Input: part model. Units: mm. Frame: model coordinates. Face numbers are marked on the shaded views. A direction names the side the tool comes from. Round coordinates to 2 decimals unless told otherwise and drop trailing zeros. Order: outer loops, then holes, each group sorted by start corner. A loop starts at its lowest first (then second) coordinate and runs counter-clockwise, first axis right, second up.
Item 1: First-contact query: pin 1 (0.9 mm diameter, centred on y = 6.5, z = 43, fed in from -X); pin 2 (2.5 mm diameter, centred on x = 0.5, z = 42.5, fed in from +Y); pin 3 (10 mm diameter, centred on x = -15, y = -23.5, fed in from +Z). Flat tips, straight axial feed; report the tip coordinate or a pass-through.
Item 2: Cut plane A-A on x = 27. Output: boundary loops of the cut face in (y, z), then the cut area to 3 significant figures.
Item 3: Cut plane B-B on y = 0. Output: boundary loops of the cut face in (x, z).
Item 4: Cut plane C-C on z = 12. Output: boundary loops of the cut face in (x, y).
Item 5: Mould query, pull axis Z, two halves, no side actions, for the marked faces 1, 2 and 3. Classes: released by +Z, released by -Z, zero draft, split by the parting line, or undercut.
Item 6: Reachability of the marked faces 4 and 5 from +Z, -Z, +X, -X, +Y, -Y: full face, straight path, thin tool, end or side. Return the list, or none.
Item 7: Cut plane D-D on y = 11. Output: boundary loops of the cut face in (x, z).
Item 8: Line query: L1, parallel to X at y = 0, z = -6.5; L2, parallel to X at y = 0, z = 31.5; L3, parallel to Y at x = 0, z = 41. Output: solid intervals per line, ascending.
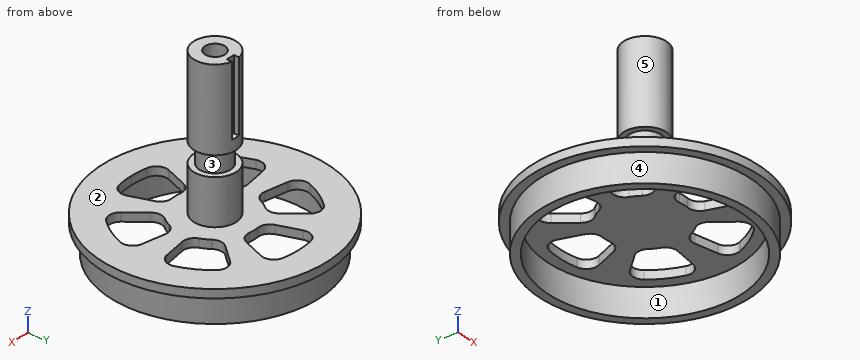
Autodesk Fusion 360 part; units mm, degrees
sketch "Sketch1" plane through (0, 0, 0) normal (0, 0, 1) x (1, 0, 0)
  circle A0 centre (0, 0) radius 33.9
  circle A1 centre (0, 0) radius 36.9
  circle A2 centre (0, 0) radius 39.9
  circle A3 centre (0, 0) radius 7.5
  circle A4 centre (0, 0) radius 14
  line L0 (0, 0) -> (4.7883, -13.1557)
  line L1 (0, 0) -> (-4.7883, -13.1557)
  line L2 (0, -60) -> (0, 60)
  line L3 (4.7883, -13.1557) -> (10.2606, -28.1908)
  line L4 (-4.7883, -13.1557) -> (-10.2606, -28.1908)
  arc A5 (10.2606, -28.1908) -> (-10.2606, -28.1908) centre (0, 0) ccw
  arc A6 (-10.2606, -28.1908) -> (0, -30) centre (0, 0) ccw
  arc A7 (0, -30) -> (10.2606, -28.1908) centre (0, 0) ccw
  line L5 (13.7873, -2.4311) -> (29.5442, -5.2094)
  line L6 (8.999, -10.7246) -> (19.2836, -22.9813)
  line L7 (8.999, 10.7246) -> (19.2836, 22.9813)
  line L8 (13.7873, 2.4311) -> (29.5442, 5.2094)
  line L9 (-4.7883, 13.1557) -> (-10.2606, 28.1908)
  line L10 (4.7883, 13.1557) -> (10.2606, 28.1908)
  line L11 (-13.7873, 2.4311) -> (-29.5442, 5.2094)
  line L12 (-8.999, 10.7246) -> (-19.2836, 22.9813)
  line L13 (-8.999, -10.7246) -> (-19.2836, -22.9813)
  line L14 (-13.7873, -2.4311) -> (-29.5442, -5.2094)
  circle A8 centre (0, 0) radius 3.5
  line L15 (-1.5, 7.3485) -> (-1.5, 5.5)
  line L16 (-1.5, 5.5) -> (1.5, 5.5)
  line L17 (1.5, 5.5) -> (1.5, 7.3485)
  circle A9 centre (0, 0) radius 5.5
  point P0 (0, 7.5)
  dimension "d1" = 67.8
  dimension "d2" = 3
  dimension "d3" = 3
  dimension "d4" = 15
  dimension "d11" = 28
  dimension "d12" = 60
  dimension "d13" = 40
  dimension "d15" = 20
  dimension "d17" = 360
  dimension "d22" = -4
  dimension "d34" = 3
  dimension "d35" = 2
  dimension "d43" = -2
extrude "Extrude1" add sketch "Sketch1" against normal blind 10 contours A0 A1 L2 | A0 A1 L2
extrude "Extrude2" add sketch "Sketch1" along normal blind 3 contours A0 L2 A5 A7 | A0 A1 L2 | A0 L2 A5 A6 | A0 A1 L2 | A4 L2 A5 L10 | A4 L2 A5 L9 | A1 A2 L2 | A1 A2 L2 | A4 L2 L4 A6 | A4 L2 L3 A7 | A3 A4 L1 L2 | A3 A4 L0 L2 | A4 A5 L7 L10 | A4 A5 L9 L12 | A3 A4 L0 L2 | A3 A4 L1 L2 | A4 L4 A5 L13 | A4 L3 A5 L6 | A4 A5 L7 L8 | A4 A5 L11 L12 | A4 A5 L13 L14 | A4 A5 L5 L6 | A4 A5 L5 L8 | A4 A5 L11 L14
extrude "Extrude3" add sketch "Sketch1" along normal blind 55 contours A3 L2 L15 L16 | A3 L2 L16 L17 | A3 L0 L2 A9 | A3 L1 L2 A9 | A3 L0 L16 L17 A9 | A3 L1 L15 L16 A9 | L0 L2 A8 A9 | L1 L2 A8 A9 | L1 L2 A8 A9 | L0 L2 A8 A9 | L0 L2 A8 | L1 L2 A8 | L1 L2 A8 | L0 L2 A8
extrude "Extrude4" cut sketch "Sketch1" along normal blind 3 contours A4 L2 A5 L10 | A4 L2 A5 L9 | A4 L2 L4 A6 | A4 L2 L3 A7 | A4 A5 L7 L8 | A4 A5 L11 L12 | A4 A5 L13 L14 | A4 A5 L5 L6
fillet "Fillet1" radius 4 24 edges at (-19.2836, 22.9813, 1.5) (-29.5442, 5.2094, 1.5) (-13.7873, 2.4311, 1.5) (-8.999, 10.7246, 1.5) (-13.7873, -2.4311, 1.5) (-29.5442, -5.2094, 1.5) (-19.2836, -22.9813, 1.5) (-8.999, -10.7246, 1.5) (-4.7883, -13.1557, 1.5) (-10.2606, -28.1908, 1.5) (10.2606, -28.1908, 1.5) (4.7883, -13.1557, 1.5) (8.999, -10.7246, 1.5) (19.2836, -22.9813, 1.5) (29.5442, -5.2094, 1.5) (13.7873, -2.4311, 1.5) (29.5442, 5.2094, 1.5) (19.2836, 22.9813, 1.5) (13.7873, 2.4311, 1.5) (8.999, 10.7246, 1.5) (4.7883, 13.1557, 1.5) (10.2606, 28.1908, 1.5) (-4.7883, 13.1557, 1.5) (-10.2606, 28.1908, 1.5)
extrude "Extrude5" cut sketch "Sketch1" against normal up to surface (52 mm away) from surface at 55 contours L0 L2 A8 | L1 L2 A8 | L1 L2 A8 | L0 L2 A8
extrude "Extrude8" cut sketch "Sketch1" against normal blind 25 from surface at 55 contours A3 L2 L15 L16 | A3 L2 L16 L17
extrude "Extrude9" cut sketch "Sketch1" along normal blind 7 from surface at 19 contours A3 L2 L15 L16 | A3 L2 L16 L17 | A3 L0 L2 A9 | A3 L1 L2 A9 | A3 L0 L16 L17 A9 | A3 L1 L15 L16 A9
From the geometry:
1. pin 1: stops at x = -4.43
1. pin 2: stops at y = 7.35
1. pin 3: stops at z = 3
2. outline: (-29.38, 0) - (-25.15, 0) - (-25.15, -10) - (-20.5, -10) - (-20.5, 0) - (-13.08, 0) - (-13.08, 3) - (-29.38, 3) - close; (-5.2, 0) - (5.2, 0) - (5.2, 3) - (-5.2, 3) - close; (13.08, 0) - (20.5, 0) - (20.5, -10) - (25.15, -10) - (25.15, 0) - (29.38, 0) - (29.38, 3) - (13.08, 3) - close
2. area: 222 mm2
3. outline: (-39.9, 0) - (-36.9, 0) - (-36.9, -10) - (-33.9, -10) - (-33.9, 0) - (33.9, 0) - (33.9, -10) - (36.9, -10) - (36.9, 0) - (39.9, 0) - (39.9, 3) - (7.5, 3) - (7.5, 19) - (5.5, 19) - (5.5, 26) - (7.5, 26) - (7.5, 55) - (3.5, 55) - (3.5, 3) - (-3.5, 3) - (-3.5, 55) - (-7.5, 55) - (-7.5, 26) - (-5.5, 26) - (-5.5, 19) - (-7.5, 19) - (-7.5, 3) - (-39.9, 3) - close
4. outline: circle Ø15 at (0, 0); hole circle Ø7 at (0, 0)
5. face 1: zero draft
5. face 2: released by +Z
5. face 3: undercut
6. face 4: -Z
6. face 5: +Z
7. outline: (-38.35, 0) - (-35.22, 0) - (-35.22, -10) - (-32.07, -10) - (-32.07, 0) - (-27.91, 0) - (-27.91, 3) - (-38.35, 3) - close; (-10.35, 0) - (10.35, 0) - (10.35, 3) - (-10.35, 3) - close; (27.91, 0) - (32.07, 0) - (32.07, -10) - (35.22, -10) - (35.22, 0) - (38.35, 0) - (38.35, 3) - (27.91, 3) - close
8. L1: x = -36.9 to -33.9, 33.9 to 36.9
8. L2: x = -7.5 to -3.5, 3.5 to 7.5
8. L3: y = -7.5 to -3.5, 3.5 to 5.5
